The model under review builds one solid part; all positions refer to its coordinate system, in mm. Coordinates: 2 decimals unless noted, no trailing zeros. Write each loop counter-clockwise with the first axis right and the second up, starting at its lowest first coordinate (ties: lowest second). Pieces come first, ordered by that corner, then holes. Notation, with made-up numbers: (85, 57) - (142, 57) arc R20 ccw to (142, 89) - close; hole circle Ø11 at (-5, -4). An arc over 180 degrees is marked (long way). Answer as CSV lines item,"result". Start each with the question number.
```python
from build123d import *

# Parameters (mm, degrees)
SKETCH1_R                        = 2.5796875
BOSS_EXTRUDE1_DEPTH              = 3.175
F_10_32_TAPPED_HOLE1_D           = 4.0386
F_10_32_TAPPED_HOLE1_CSINK_D     = 6.096
F_10_32_TAPPED_HOLE1_CSINK_ANGLE = 90


with BuildPart() as part:
    # Sketch1 → Boss-Extrude1 (new body)
    with BuildSketch(Plane(origin=(0, 0, 0), x_dir=(1, 0, 0), z_dir=(0, 1, 0))):
        with BuildLine():
            Line((-95.25, 6.35), (95.25, 6.35))
            ThreePointArc((95.25, 6.35), (101.6, 0), (95.25, -6.35))
            Line((95.25, -6.35), (-95.25, -6.35))
            ThreePointArc((-95.25, -6.35), (-101.6, 0), (-95.25, 6.35))
        make_face()
        with Locations((95.25, 0)):
            Circle(SKETCH1_R, mode=Mode.SUBTRACT)
        with Locations((-95.25, 0)):
            Circle(SKETCH1_R, mode=Mode.SUBTRACT)
        Circle(SKETCH1_R, mode=Mode.SUBTRACT)
    extrude(amount=BOSS_EXTRUDE1_DEPTH)

    # #10-32 Tapped Hole1 (through all)
    with Locations(Plane(origin=(0, 3.175, 0), x_dir=(1, 0, 0), z_dir=(0, 1, 0))):
        with Locations((-95.25, 0), (0, 0), (95.25, 0)):
            CounterSinkHole(F_10_32_TAPPED_HOLE1_D / 2, F_10_32_TAPPED_HOLE1_CSINK_D / 2, counter_sink_angle=F_10_32_TAPPED_HOLE1_CSINK_ANGLE)


solid = part.part
```
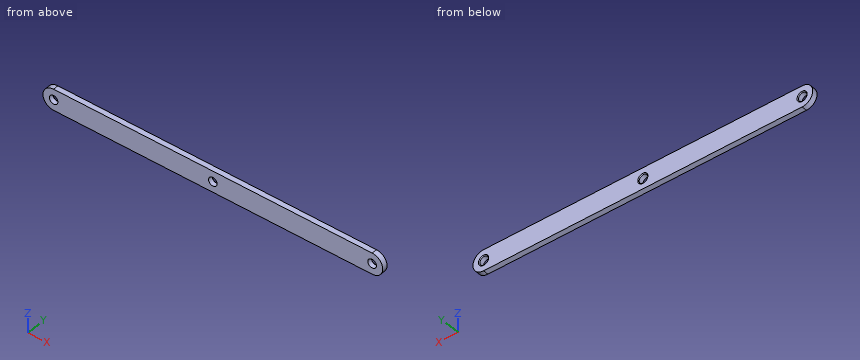
(1) Add section B-B on x = 0. Give the boundary of the cut face in (y, z) (3 decimals), then the cut area to 3 significant figures.
(2) Add section C-C on z = 0. Give the boundary of the cut face in (x, y) (3 decimals), then the cut area to 3 significant figures.
(3) Add section A-A on y = 1.1. Give the boundary of the cut face in (x, z), then the cut area to 3 significant figures.
(4) Wall thickness on line 1 (X direction, y = 1.3, z = 0); line 2 (Z direction, x = 95.25, y = 1.75); line 3 (X direction, y = 2.85, z = 1.25): over which ranges is each line inside the solid? List them lowest first.
Reported:
1,outline,"(0, -6.35) - (3.175, -6.35) - (3.175, -3.048) - (2.707, -2.58) - (0, -2.58) - close; (0, 2.58) - (2.707, 2.58) - (3.175, 3.048) - (3.175, 6.35) - (0, 6.35) - close"
1,area,"23.7 mm²"
2,outline,"(-101.6, 0) - (-97.83, 0) - (-97.83, 2.707) - (-98.298, 3.175) - (-101.6, 3.175) - close; (-92.67, 0) - (-2.58, 0) - (-2.58, 2.707) - (-3.048, 3.175) - (-92.202, 3.175) - (-92.67, 2.707) - close; (2.58, 0) - (92.67, 0) - (92.67, 2.707) - (92.202, 3.175) - (3.048, 3.175) - (2.58, 2.707) - close; (97.83, 0) - (101.6, 0) - (101.6, 3.175) - (98.298, 3.175) - (97.83, 2.707) - close"
2,area,"595 mm²"
3,outline,"(-95.25, -6.35) - (95.25, -6.35) arc R6.35 ccw to (95.25, 6.35) - (-95.25, 6.35) arc R6.35 ccw to start; hole circle Ø5.16 at (-95.25, 0); hole circle Ø5.16 at (0, 0); hole circle Ø5.16 at (95.25, 0)"
3,area,"2,480 mm²"
4,line 1,"-101.6 to -97.83, -92.67 to -2.58, 2.58 to 92.67, 97.83 to 101.6"
4,line 2,"-6.35 to -2.58, 2.58 to 6.35"
4,line 3,"-101.48 to -97.67, -92.83 to -2.42, 2.42 to 92.83, 97.67 to 101.48"
